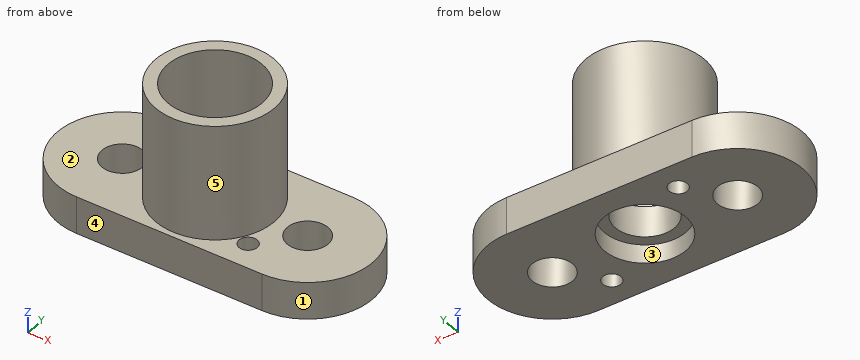
```python
from build123d import *

# Parameters (mm, degrees)
F0_R     = 0.4935
F0_R_2   = 1.1
F1_DEPTH = 2
F2_R     = 3.2
F3_DEPTH = 0.65
F4_R     = 3.2
F4_R_2   = 2.5375
F5_DEPTH = 5.55
F6_R     = 1.6
F7_DEPTH = 25
F8_R     = 2.2
F9_DEPTH = 1


with BuildPart() as f1:
    # F0 (on Top) → F1 (new body)
    with BuildSketch(Plane.XY):
        with BuildLine():
            Line((5, 3.5), (-5, 3.5))
            ThreePointArc((-5, 3.5), (-8.5, 0), (-5, -3.5))
            Line((-5, -3.5), (5, -3.5))
            ThreePointArc((5, -3.5), (8.5, 0), (5, 3.5))
        make_face()
        with Locations((3.2, -2)):
            Circle(F0_R, mode=Mode.SUBTRACT)
        with Locations((-5, 0)):
            Circle(F0_R_2, mode=Mode.SUBTRACT)
        with Locations((-3.2, 2)):
            Circle(F0_R, mode=Mode.SUBTRACT)
        with Locations((5, 0)):
            Circle(F0_R_2, mode=Mode.SUBTRACT)
    extrude(amount=F1_DEPTH)

    # F2 (on face) → F3 (join)
    with BuildSketch(Plane.XY.offset(2)):
        Circle(F2_R)
    extrude(amount=F3_DEPTH)

    # F4 (on face) → F5 (join)
    with BuildSketch(Plane.XY.offset(2.65)):
        Circle(F4_R)
        Circle(F4_R_2, mode=Mode.SUBTRACT)
    extrude(amount=F5_DEPTH)

    # F6 (on face) → F7 (cut)
    with BuildSketch(Plane.XY.offset(2.65)):
        Circle(F6_R)
    extrude(amount=-F7_DEPTH, mode=Mode.SUBTRACT)

    # F8 (on face) → F9 (cut)
    with BuildSketch(Plane(origin=(0, 0, 0), x_dir=(1, 0, 0), z_dir=(0, 0, -1))):
        Circle(F8_R)
    extrude(amount=-F9_DEPTH, mode=Mode.SUBTRACT)


solid = f1.part
```
The listing builds one solid part. Answer for the finished solid, in the listing's coordinates (mm). Face numbers are marked on the shaded views. A direction names the side the tool comes from. Give positions to 0.01 mm unless a question says otherwise; leave off trailing zeros. Loops run counter-clockwise (first coordinate to the right, second up) from the corner with the lowest first, then second, coordinate; pieces in that order, holes last. Notation, with made-up numbers: M -37.75,-23 L 2.25,-23 A23 cw 2.25,-5 Z; hole C 67,19.25 d8. An arc over 180 degrees is marked long. One line per item, written item: value.
1. For the marked faces 4 and 5, determine the directions among +Z, -Z, +X, -X, +Y, -Y from which every point of the face is accessible in a straight line to the end or side of a thin tool.
Found:
face 4: +Z, -Z, +X, -X, -Y
face 5: +Z
2. Section A-A on x = 0.25 is taken. Determine the outline of the cut face in (y, z), plus the area to 3 significant figures.
Found:
outline: M -3.5,0 L -2.19,0 L -2.19,1 L -1.58,1 L -1.58,2.65 L -2.53,2.65 L -2.53,8.2 L -3.19,8.2 L -3.19,2 L -3.5,2 Z; M 1.58,1 L 2.19,1 L 2.19,0 L 3.5,0 L 3.5,2 L 3.19,2 L 3.19,8.2 L 2.53,8.2 L 2.53,2.65 L 1.58,2.65 Z
area: 15.9 mm^2
3. Find the intervals of material crossed by probe 1 along Y at (x, z) = (0, 2.2); probe 2 along Z at (x, y) = (4.75, -2.5); probe 3 along Y at (x, z) = (0, 4.85), in increasing order.
Found:
probe 1: -3.2 to -1.6, 1.6 to 3.2
probe 2: 0 to 2
probe 3: -3.2 to -2.54, 2.54 to 3.2
4. Each of these flat-tipped pins is pushed along its axis until it touches: P1, Ø3.5, axis at x = 0, y = 0, coming from the +Z side; P2, Ø2, axis at x = 5, y = 0, coming from the -Z side; P3, Ø4, axis at x = -3.5, z = 7, coming from the +Y side; P4, Ø3.5, axis at x = -5, y = 0, coming from the +Z side. Where does it stop, or does it pass through?
Found:
P1: z = 2.65
P2: through
P3: y = 2.83
P4: z = 2
5. Section B-B on y = -0.5 is taken. Determine the outline of the cut face in (x, z).
Found:
outline: M -8.46,0 L -5.98,0 L -5.98,2 L -8.46,2 Z; M -4.02,0 L -2.14,0 L -2.14,1 L -1.52,1 L -1.52,2.65 L -2.49,2.65 L -2.49,8.2 L -3.16,8.2 L -3.16,2 L -4.02,2 Z; M 1.52,1 L 2.14,1 L 2.14,0 L 4.02,0 L 4.02,2 L 3.16,2 L 3.16,8.2 L 2.49,8.2 L 2.49,2.65 L 1.52,2.65 Z; M 5.98,0 L 8.46,0 L 8.46,2 L 5.98,2 Z
6. Section D-D on y = 2 is taken. Determine the outline of the cut face in (x, z), plus the area to 3 significant figures.
Found:
outline: M -7.87,0 L -3.69,0 L -3.69,2 L -7.87,2 Z; M -2.71,0 L -0.92,0 L -0.92,1 L 0.92,1 L 0.92,0 L 7.87,0 L 7.87,2 L 2.5,2 L 2.5,8.2 L 1.56,8.2 L 1.56,2.65 L -1.56,2.65 L -1.56,8.2 L -2.5,8.2 L -2.5,2 L -2.71,2 Z
area: 41.3 mm^2
7. For a pull along Y with two mould halves and no side action, classify the marked faces 1, 2 and 3 as pulls with the +Y half, pulls with the -Y half, needs draft (parallel to the pull), parting line crosses it, or undercut.
Found:
face 1: parting line crosses it
face 2: needs draft
face 3: undercut
8. Section C-C on z = 5 is taken. Determine the outline of the cut face in (x, y) (1 decimal), plus the area to 3 significant figures.
Found:
outline: C 0,0 d6.4; hole C 0,0 d5.1
area: 11.9 mm^2
